Geometry check sheet. Reference: the model listing, model coordinates, mm. A direction names the side the tool comes from. Give positions to 0.01 mm unless a question says otherwise; leave off trailing zeros. Write each loop counter-clockwise with the first axis right and the second up, starting at its lowest first coordinate (ties: lowest second). Pieces come first, ordered by that corner, then holes. Notation, with made-up numbers: (-9, 79) - (20, 79) arc R8 ccw to (20, 83) - close; hole circle Ø3 at (7.5, 60). An arc over 180 degrees is marked (long way). Use a Markdown table: item, result.
```python
from build123d import *

# Parameters (mm, degrees)
FILLET1_R   = 0.1
HEX_2_DEPTH = 1.2


with BuildPart() as part:
    # BodySke → BaseBody (revolve)
    with BuildSketch(Plane.XY):
        Polygon((0, 0), (0, 2.85), (0.35, 2.85), (1.7, 1.5), (9.7195, 1.5), (10, 1.2195), (10, 0), align=None)
    revolve(axis=Axis((0, 0, 0), (1, 0, 0)))

    # Fillet1
    fillet1_edges = [part.edges().sort_by_distance(p)[0] for p in [
        (1.7, -1.5, 0),
    ]]
    fillet(fillet1_edges, radius=FILLET1_R)

    # Sketch2 → PreBroach (revolve, cut)
    with BuildSketch(Plane.XY):
        Polygon((0, 1.01), (1.2, 1.01), (1.783123772, 0), (0, 0), align=None)
    revolve(axis=Axis((0, 0, 0), (1, 0, 0)), mode=Mode.SUBTRACT)

    # Sketch3 → Hex 2 (cut)
    with BuildSketch(Plane.ZY):
        Polygon((-1.01, -0.583123772), (-1.01, 0.583123772), (0, 1.166247544), (1.01, 0.583123772), (1.01, -0.583123772), (0, -1.166247544), align=None)
    extrude(amount=-HEX_2_DEPTH, mode=Mode.SUBTRACT)


solid = part.part
```
1) Mould release check, pull along Y, two halves, no side actions. Record for faces 1 (the flat face through (0.592, -0.879, -0.498)), 2 (the cylindrical face through (5.79, -1.5, 0.07)), 3 (the flat face through (1, 0, -1.01)), 4 (the flat face through (10, 0, 0)): pulls with the +Y half, pulls with the -Y half, needs draft (parallel to the pull), parting line crosses it, or undercut.
Working result:
| item | result |
|---|---|
| face 1 | undercut |
| face 2 | parting line crosses it |
| face 3 | undercut |
| face 4 | needs draft |
2) Set-up check for faces 5 (the flat face through (0.592, 0.879, 0.498)), 6 (the flat face through (0, 0, -1.2)): record each of +Z, -Z, +X, -X, +Y, -Y from which the full face is reachable in a straight line by a thin tool's end or side.
Working result:
| item | result |
|---|---|
| face 5 | -X |
| face 6 | +Z, -Z, -X, +Y, -Y |
3) Material ranges on L1, parallel to Y at x = 6.75, z = -0.1; L2, parallel to Y at x = 1.25, z = -0.05; L3, parallel to Z at x = 7.5, y = 0.55, recorded low to high. Write a range as from..to.
Working result:
| item | result |
|---|---|
| L1 | y = -1.5..1.5 |
| L2 | y = -1.95..-0.92, 0.92..1.95 |
| L3 | z = -1.4..1.4 |
4) Section check A-A on x = 5.25. Record the boundary of the cut face in (y, z), then the cut area to 3 significant figures.
Working result:
| item | result |
|---|---|
| outline | circle Ø3 at (0, 0) |
| area | 7.07 mm² |
5) Depth check by flat-ended pin: P1, Ø3, axis at y = -1.5, z = -1.5, coming from the +X side; P2, Ø1.5, axis at x = 4.5, y = 1, coming from the +Z side; P3, Ø3, axis at x = 8.5, z = -2, coming from the +Y side. Enter the tip coordinate at first touch or a pass-through.
Working result:
| item | result |
|---|---|
| P1 | stops at x = 10 |
| P2 | stops at z = 1.48 |
| P3 | stops at y = 1.41 |
